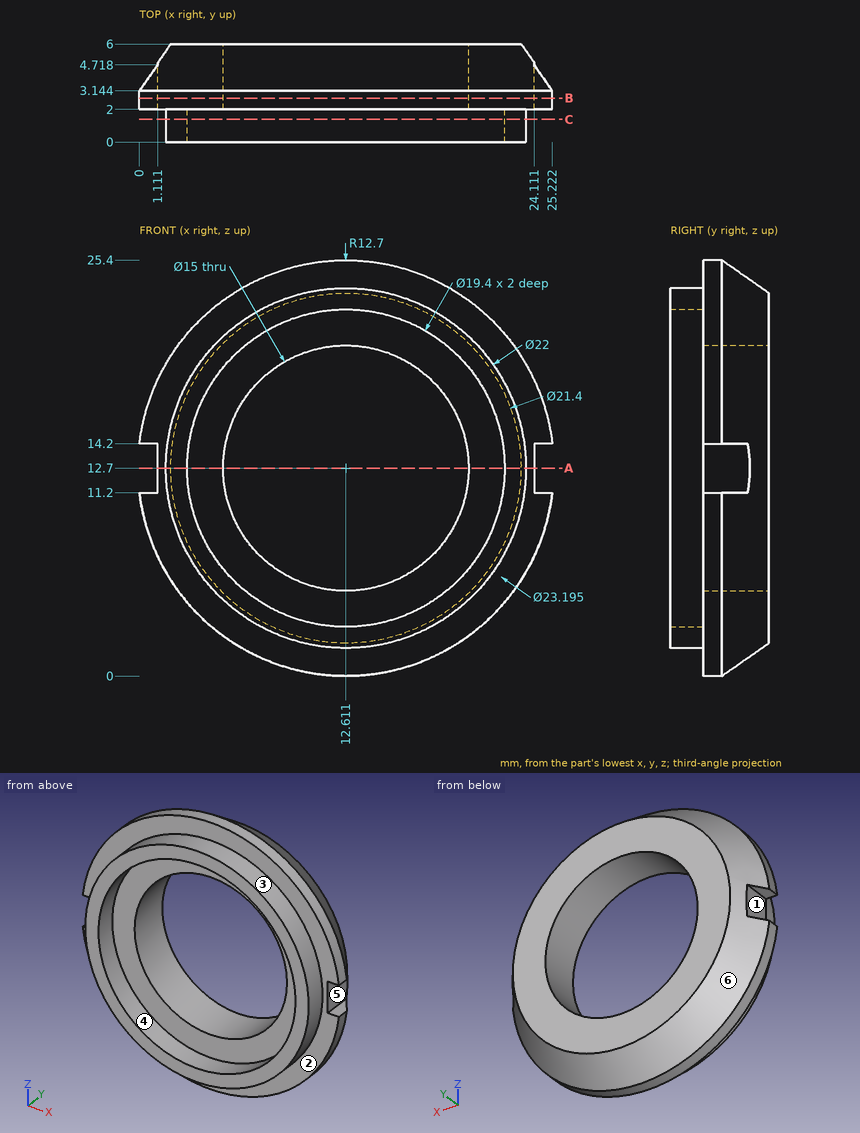
Design review of the part shown in the three views and the two pictorial views. Dimensions are in mm from the part's minimum x, y and z. A direction names the side the tool comes from. Round coordinates to 2 decimals unless told otherwise and drop trailing zeros. Loops run counter-clockwise (first coordinate to the right, second up) from the corner with the lowest first, then second, coordinate; pieces in that order, holes last. Notation, with made-up numbers: M 68,65 L 113,65 A16 cw 113,78 Z; hole C -22,36 d11. An arc over 180 degrees is marked long. Answer as a JSON object with one key per item and string values.
Item 1: Wall thickness on L1, parallel to X at y = 1.1, z = 12.7; L2, parallel to X at y = 3, z = 12.7; L3, parallel to Y at x = 9.75, z = 4: over which ranges is each line inside the solid? List them lowest first. Write a range as from..to.
Answer sheet:
{"L1": "x = 1.61..2.91, 22.31..23.61", "L2": "x = 1.11..5.11, 20.11..24.11", "L3": "y = 2..6"}
Item 2: The part is to be moulded in two halves that separate along Z. For the marked faces 1, 2 and 3, say which applies: pulls with the +Z half, pulls with the -Z half, needs draft (parallel to the pull), parting line crosses it, or undercut.
Answer sheet:
{"face 1": "undercut", "face 2": "needs draft", "face 3": "parting line crosses it"}
Item 3: We need section C-C on y = 1.4. Give the boundary of the cut face in (x, z).
Answer sheet:
{"outline": "C 12.61,12.7 d22; hole C 12.61,12.7 d19.4"}
Item 4: Machinability: for the marked faces 4, 5 and 6, which of the approach directions +Z, -Z, +X, -X, +Y, -Y give a long, thin tool a straight path to every point of the face, cutting with its end or side? Answer none if there is none.
Answer sheet:
{"face 4": "-Y", "face 5": "+X, +Y, -Y", "face 6": "+Y"}
Item 5: We need section A-A on z = 12.7. Give the boundary of the cut face in (x, y).
Answer sheet:
{"outline": "M 1.11,2 L 1.61,2 L 1.61,0 L 2.91,0 L 2.91,2 L 5.11,2 L 5.11,6 L 1.91,6 L 1.11,4.86 Z; M 20.11,2 L 22.31,2 L 22.31,0 L 23.61,0 L 23.61,2 L 24.11,2 L 24.11,4.86 L 23.31,6 L 20.11,6 Z"}
Item 6: We need section B-B on y = 2.7. Give the boundary of the cut face in (x, z).
Answer sheet:
{"outline": "M 0,11.2 A12.7 ccw 25.22,11.2 L 24.11,11.2 L 24.11,14.2 L 25.22,14.2 A12.7 ccw 0,14.2 L 1.11,14.2 L 1.11,11.2 Z; hole C 12.61,12.7 d15"}
Item 7: Clearance check with flat-ended pins moving along their axes: P1, Ø3, axis at y = 5, z = 20.5, coming from the +X side; P2, Ø3, axis at x = 11.5, z = 19.5, coming from the -Y side; P3, Ø2, axis at x = 2.5, y = 2, coming from the +Z side. State where each tip first meets the part, or that it passes through.
Answer sheet:
{"P1": "stops at x = 22.72", "P2": "stops at y = 2", "P3": "stops at z = 21.55"}
